Geometry check sheet. Reference: the model listing, model coordinates, mm. A direction names the side the tool comes from. Give positions to 0.01 mm unless a question says otherwise; leave off trailing zeros. Write each loop counter-clockwise with the first axis right and the second up, starting at its lowest first coordinate (ties: lowest second). Pieces come first, ordered by that corner, then holes.
(1) Cross-section at C-C (z = -6.35). Record the boundary of the cut face in (x, y).
(2) Thickness scan on line 1 along Z through (x, y) = (6.35, -5.5); line 2 along X through (y, z) = (-4.5, -7.5); line 3 along X through (y, z) = (-4.75, -6). Record the ranges inside material, lowest first.
(3) Depth check by flat-ended pin: P1, Ø4, axis at y = -8, z = -8, coming from the -X side; P2, Ø1.5, axis at y = -6.5, z = -11.5, coming from the -X side; P3, Ø3, axis at x = 6.35, z = -6.35, coming from the +Y side; P4, Ø0.5, axis at x = 46.5, y = -9.5, coming from the -Z side. Enter the tip coordinate at first touch or a pass-through.
(4) Cross-section at D-D (x = 35.5). Record the boundary of the cut face in (y, z), and give its area (3 significant figures).
(5) Tool access check on faces 5 (the cylindrical face through (45.15, -6.26, -2.76)), 6 (the flat face through (46.4, -6.3, -9.652)), 7 (the cylindrical face through (56.02, -6.44, -0.48)). Record the directions out of +Z, -Z, +X, -X, +Y, -Y that give a thin tool (end or side, any length) a straight path to the whole face; none if there is none.
(6) Cross-section at B-B (x = 6.35). Record the boundary of the cut face in (y, z), and give its area (3 significant figures).
(7) Mould release check, pull along X, two halves, no side actions. Record for faces 1 (the cylindrical face through (47.456, -6.439, -9.528)), 2 (the cylindrical face through (11.172, -6.439, -11.251)), 3 (the flat face through (0, -6, -6)), 4 (the flat face through (6, -6, -12.7)): +X half, -X half, draft (parallel to the pull), parting line (faces both ways), or undercut.
```python
from build123d import *

# Parameters (mm, degrees)
F0_R     = 1.778
F1_DEPTH = 12.7
F2_R     = 1.5875
F3_R     = 0.762
F4_R     = 5.08


with BuildPart() as f1:
    # F0 (on Front) → F1 (new body)
    with BuildSketch(Plane.XZ):
        with BuildLine():
            Line((57.15, 0), (0, 0))
            Line((0, 0), (0, -12.7))
            Line((0, -12.7), (12.7, -12.7))
            Line((12.7, -12.7), (12.7, -4.572))
            ThreePointArc((12.7, -4.572), (13.443949, -2.775949), (15.24, -2.032))
            Line((15.24, -2.032), (43.3705, -2.032))
            ThreePointArc((43.3705, -2.032), (45.166551, -2.775949), (45.9105, -4.572))
            Line((45.9105, -4.572), (45.9105, -9.652))
            Line((45.9105, -9.652), (47.498, -9.652))
            Line((47.498, -9.652), (57.15, 0))
        make_face()
        with Locations((6.35, -6.35)):
            Circle(F0_R, mode=Mode.SUBTRACT)
    extrude(amount=F1_DEPTH)

    # F2
    f2_edges = [f1.edges().sort_by_distance(p)[0] for p in [
        (47.498, -6.35, -9.652),
    ]]
    fillet(f2_edges, radius=F2_R)

    # F3
    f3_edges = [f1.edges().sort_by_distance(p)[0] for p in [
        (57.15, -6.35, 0),
    ]]
    fillet(f3_edges, radius=F3_R)

    # F4
    f4_edges = [f1.edges().sort_by_distance(p)[0] for p in [
        (0, -6.35, -12.7),
        (12.7, -6.35, -12.7),
        (0, -6.35, 0),
    ]]
    fillet(f4_edges, radius=F4_R)


solid = f1.part
```
Reply:
1. outline: (0, -12.7) - (4.57, -12.7) - (4.57, 0) - (0, 0) - close; (8.13, -12.7) - (12.7, -12.7) - (12.7, 0) - (8.13, 0) - close; (45.91, -12.7) - (50.8, -12.7) - (50.8, 0) - (45.91, 0) - close
2. line 1: z = -12.7 to -8.13, -4.57 to 0
2. line 2: x = 0 to 4.99, 7.71 to 12.7, 45.91 to 49.65
2. line 3: x = 0 to 4.61, 8.09 to 12.7, 45.91 to 51.15
3. P1: stops at x = 0
3. P2: stops at x = 1.08
3. P3: passes through
3. P4: stops at z = -9.65
4. outline: (-12.7, -2.03) - (0, -2.03) - (0, 0) - (-12.7, 0) - close
4. area: 25.8 mm2
5. face 5: -Z, +Y, -Y
5. face 6: -Z, +X, +Y, -Y
5. face 7: +X, +Y, -Y
6. outline: (-12.7, -12.7) - (0, -12.7) - (0, -8.13) - (-12.7, -8.13) - close; (-12.7, -4.57) - (0, -4.57) - (0, 0) - (-12.7, 0) - close
6. area: 116 mm2
7. face 1: +X half
7. face 2: undercut
7. face 3: -X half
7. face 4: draft
